Study the drawing (mm; zero at the part's minimum x, y, z) and answer. A direction names the side the tool comes from. Round coordinates to 2 decimals unless told otherwise and drop trailing zeros.
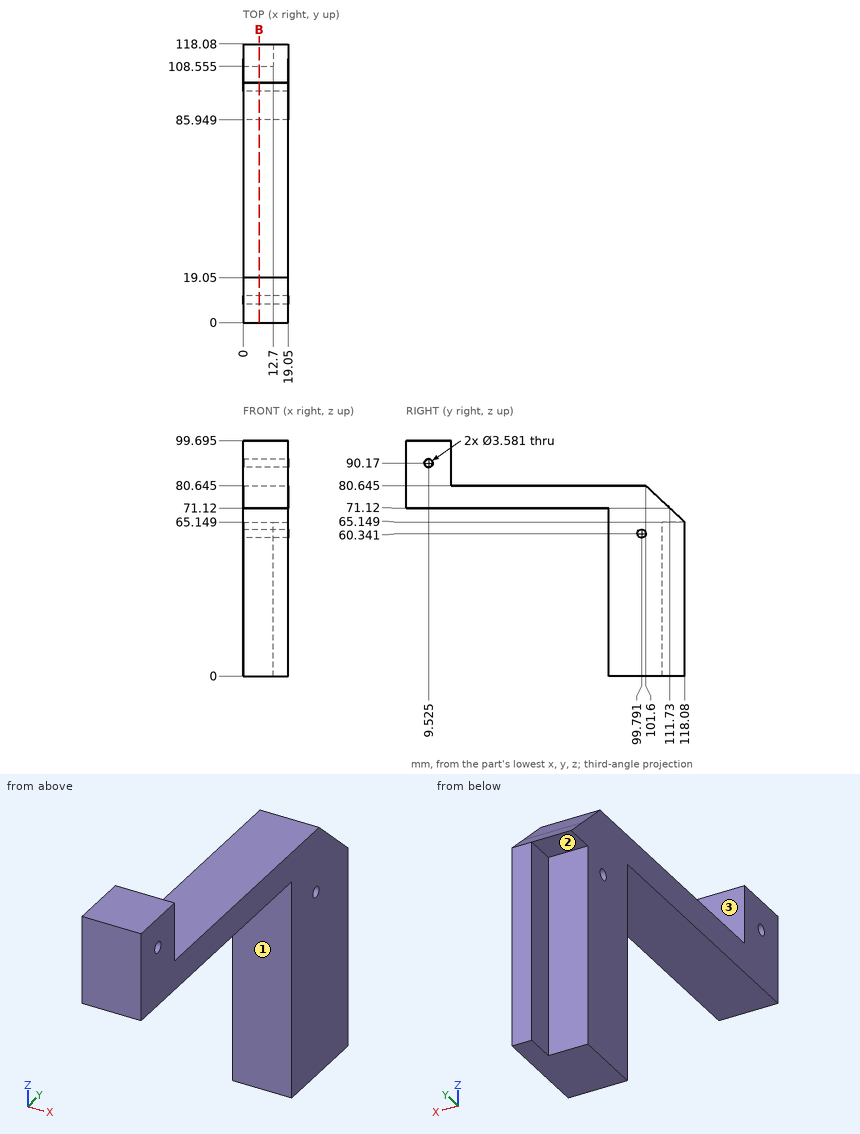
1. Straight lines are drawn through the part: line 1 along Z through (x, y) = (2, 100) (1 decimal); line 2 along Z through (x, y) = (5.5, 73) (1 decimal); line 3 along Y through (x, z) = (14.75, 35.5). For each, find the intervals that lie inside material, in ascending order.
Geometry says:
line 1: z = 0 to 58.6, 62.1 to 80.6
line 2: z = 71.1 to 80.6
line 3: y = 85.95 to 118.08
2. Given pin 1 (2 mm diameter, centred on x = 3.5, y = 56.5, fed in from -Z); pin 2 (1.5 mm diameter, centred on x = 15.5, y = 101, fed in from +Z) (1 decimal); pin 3 (7.5 mm diameter, centred on y = 115.5, z = 48.5, fed in from -X); pin 4 (3 mm diameter, centred on y = 99.79, z = 60.34, fed in from +X), each flat-ended and moving along its own axis, determine where each tip first touches the part or whether it passes through.
Geometry says:
pin 1: stops at z = 71.12
pin 2: stops at z = 80.6
pin 3: stops at x = 12.7
pin 4: passes through
3. A tool of negligible diameter and unlimited length cuts with its end or side. For the marked faces 1, 2 and 3, from which of +Z, -Z, +X, -X, +Y, -Y can it reach the whole face along a straight path? Write none if from no direction.
Geometry says:
face 1: -Z, +X, -X, -Y
face 2: -Z, -X, +Y
face 3: +Z, +X, -X, +Y
4. Section B-B on x = 6.75 is taken. Give the number of separate pieces and of enclosed holes in the cut face, plus the area to 3 significant figures.
Geometry says:
separate pieces: 1
enclosed holes: 2
area: 3,000 mm2
